Autodesk Inventor part; units mm, degrees
ref_plane "YZ Plane" through (0, 0, 0) normal (1, 0, 0) x (0, 1, 0)
ref_plane "XZ Plane" through (0, 0, 0) normal (0, 1, 0) x (-1, 0, 0)
ref_plane "XY Plane" through (0, 0, 0) normal (0, 0, 1) x (1, 0, 0)
sketch "Sketch1" plane through (0, 0, 0) normal (0, 1, 0) x (-1, 0, 0)
  circle A0 centre (0, 0) radius 12
  circle A1 centre (-0.0043, 0) radius 3.75
  circle A2 centre (-0.0043, 0) radius 6.375 construction
  circle A3 centre (-0.0043, 0) radius 9.375 construction
  circle A4 centre (-0.0043, 0) radius 7.875 construction
  circle A5 centre (0, -7.875) radius 0.6
  circle A6 centre (6.3707, 0) radius 0.6
  circle A7 centre (9.3707, 0) radius 0.6
  line L0 (16.292, 0) -> (-19, 0) construction
  line L1 (0, 21) -> (0, -27.3544) construction
  circle A8 centre (0, 7.875) radius 0.6
  circle A9 centre (-6.3707, 0) radius 0.6
  circle A10 centre (-9.3707, 0) radius 0.6
  line L2 (-0.0043, 0) -> (-8.4874, 8.4831) construction
  line L3 (-0.0043, 0) -> (11.9927, 0) construction
  circle A11 centre (-5.5728, 5.5685) radius 1
  circle A12 centre (5.5728, 5.5685) radius 1
  circle A13 centre (-5.5728, -5.5685) radius 1
  circle A14 centre (5.5728, -5.5685) radius 1
  circle A15 centre (-2.4685, 7.4795) radius 0.6
  circle A16 centre (2.4685, 7.4795) radius 0.6
  circle A17 centre (-2.4685, -7.4795) radius 0.6
  circle A18 centre (2.4685, -7.4795) radius 0.6
  circle A19 centre (6.057, 1.9752) radius 0.6
  circle A20 centre (8.8907, 2.9614) radius 0.6
  circle A21 centre (6.057, -1.9752) radius 0.6
  circle A22 centre (8.8907, -2.9614) radius 0.6
  circle A23 centre (-6.057, 1.9752) radius 0.6
  circle A24 centre (-8.8907, 2.9614) radius 0.6
  circle A25 centre (-8.8907, -2.9614) radius 0.6
  circle A26 centre (-6.057, -1.9752) radius 0.6
  dimension "d4" = 24
  dimension "d2" = 7.5
  dimension "d6" = 12.75
  dimension "d7" = 18.75
  dimension "d8" = 15.75
  dimension "d9" = 1.2
  dimension "d13" = 1.2
  dimension "d14" = 1.2
  dimension "d27" = 135
  dimension "d29" = 1.2
  dimension "d33" = 1.3
  dimension "d34" = 2
  dimension "d35" = 0.8
  dimension "d36" = 1.2
  dimension "d37" = 1.2
  dimension "d38" = 1.8
extrude "Extrusion4" add sketch "Sketch1" along normal blind 6.5 contours A0 | A11 | A12 | A13 | A14
extrude "Extrusion5" add sketch "Sketch1" along normal blind 3.5 contours A5 | A6 | A7 | A8 | A9 | A10 | A15 | A16 | A17 | A18 | A19 | A20 | A21 | A22 | A23 | A24 | A25 | A26
extrude "Extrusion6" cut sketch "Sketch1" along normal blind 4 contours A11 | A12 | A13 | A14
equation "\"d13\" = d9"
equation "\"d14\" = d9"
equation "\"d29\" = d9"
equation "\"d36\" = d13"
equation "\"d37\" = d14"
properties part number "engine_connector_sleeve"
The listing builds one solid part. Answer for the finished solid, in the listing's coordinates (mm). A direction names the side the tool comes from. Give positions to 0.01 mm unless a question says otherwise; leave off trailing zeros. Loops run counter-clockwise (first coordinate to the right, second up) from the corner with the lowest first, then second, coordinate; pieces in that order, holes last. Notation, with made-up numbers: (58.25, 54) - (67.25, 54) arc R12 ccw to (67.25, 61) - close; hole circle Ø8 at (43, 5). An arc over 180 degrees is marked (long way). Write each question's results on one line, items separated by ' | '.
1. Find section C-C, the plane y = 5. Count the separate pieces of the cut face and the enclosed holes in it, then the cut area to 3 significant figures.
Resolved:
separate pieces: 1 | enclosed holes: 19 | area: 388 mm^2
2. Find section A-A, the plane z = 0. Write down the section's boundary in (x, y).
Resolved:
outline: (-12, 0) - (-3.75, 0) - (-3.75, 6.5) - (-5.77, 6.5) - (-5.77, 3.5) - (-6.97, 3.5) - (-6.97, 6.5) - (-8.77, 6.5) - (-8.77, 3.5) - (-9.97, 3.5) - (-9.97, 6.5) - (-12, 6.5) - close; (3.75, 0) - (12, 0) - (12, 6.5) - (9.97, 6.5) - (9.97, 3.5) - (8.77, 3.5) - (8.77, 6.5) - (6.97, 6.5) - (6.97, 3.5) - (5.77, 3.5) - (5.77, 6.5) - (3.75, 6.5) - close
3. Which of the six approach directions +Z, -Z, +X, -X, +Y, -Y give full straight-line access (tool end or side, diameter ignored) to faces 1 (the face through (-3.57, 3.2, -1.13)), 2 (the face through (6, 3.5, -2)), 3 (the face through (5.035, 1.972, -6.412))?
Resolved:
face 1: +Y, -Y | face 2: +Y | face 3: -Y
4. Flat-ended cylindrical pins translate along their axes: P1, Ø1.1, axis at x = 2.47, z = 7.48, coming from the +Y side; P2, Ø1, axis at x = -2, y = 1, coming from the +Z side; P3, Ø1.5, axis at y = 5, z = 8, coming from the +X side. Find the tip coordinate at first contact, or state that the pin passes through.
Resolved:
P1: stops at y = 3.5 | P2: stops at z = 11.91 | P3: stops at x = 9.56
5. Find section D-D, the plane y = 2.75. Write down the section's boundary in (x, z).
Resolved:
outline: circle Ø24 at (0, 0); hole circle Ø2 at (-5.57, -5.57); hole circle Ø2 at (-5.57, 5.57); hole circle Ø7.5 at (0, 0); hole circle Ø2 at (5.57, -5.57); hole circle Ø2 at (5.57, 5.57)
6. Find section B-B, the plane x = 0. Write down the section's boundary in (y, z) (3 decimals).
Resolved:
outline: (0, -12) - (6.5, -12) - (6.5, -8.475) - (3.5, -8.475) - (3.5, -7.275) - (6.5, -7.275) - (6.5, -3.75) - (0, -3.75) - close; (0, 3.75) - (6.5, 3.75) - (6.5, 7.275) - (3.5, 7.275) - (3.5, 8.475) - (6.5, 8.475) - (6.5, 12) - (0, 12) - close
7. Consider probe 1 along Z at (x, y) = (3, 4.25); probe 2 along X at (y, z) = (3.75, -2.5); probe 3 along X at (y, z) = (0.75, -5.5). Determine where each line is inside the solid, lowest interval first. Write a range as from..to.
Resolved:
probe 1: z = -11.62..-7.76, -7.2..-2.26, 2.26..7.2, 7.76..11.62 | probe 2: x = -11.74..-9.27, -8.51..-6.35, -5.77..-2.79, 2.8..5.77, 6.35..8.51, 9.27..11.74 | probe 3: x = -10.67..-6.57, -4.58..4.58, 6.57..10.67
